```python
from build123d import *

# Parameters (mm, degrees)
F1_R   = 13.7541
F1_R_2 = 10.6807


with BuildPart() as f3:
    # F3: sweep along a path in F2
    with BuildLine(Plane.XY) as f3_path:
        Line((45.4025, 13.7541), (25.0317, 13.7541))
        ThreePointArc((25.0317, 13.7541), (7.3316151854, 6.4224848146), (0, -11.2776))
        Line((0, -11.2776), (0, -31.6484))
    # F1 (on offset) → F3 (sweep)
    with BuildSketch(Plane.XZ.offset(31.6484)):
        Circle(F1_R)
        Circle(F1_R_2, mode=Mode.SUBTRACT)
    sweep(path=f3_path.line)


solid = f3.part
```
Check sheet for the modelled part. Datum: model origin and axes. Units: mm. A direction names the side the tool comes from. Coordinates: 2 decimals unless noted, no trailing zeros. Write each loop counter-clockwise with the first axis right and the second up, starting at its lowest first coordinate (ties: lowest second). Pieces come first, ordered by that corner, then holes. Notation, with made-up numbers: M 15,3 L 31,3 A32 cw 31,29 Z; hole C 29.25,77.25 d8. An arc over 180 degrees is marked long. Write item = value, one per line. Start each with the question number.
1. Sectioned sample at C-C (y = -22). Record the cut outline in (x, z), then the cut area to 3 significant figures.
2. Sectioned sample at A-A (z = 0). Record the cut outline in (x, y), then the cut area to 3 significant figures.
3. Tool access check on faces 4 (the cylindrical face through (9.866, -21.606, -4.091)), 5 (the flat face through (-7.1, -31.648, 8.2)), 6 (the cylindrical face through (35.075, 0.635, 4.131)). Record the directions out of +Z, -Z, +X, -X, +Y, -Y that give a thin tool (end or side, any length) a straight path to the whole face; none if there is none.
4. Sectioned sample at D-D (z = -3.5). Record the cut outline in (x, y).
5. Thickness scan on probe 1 along Z at (x, y) = (0, -26.5); probe 2 along Z at (x, y) = (12.5, 11); probe 3 along Y at (x, z) = (29.5, -5.75). Record the ranges inside material, lowest first.
6. Go/stop test with flat-tipped pins: pin 1 (1 mm diameter, centred on y = 11, z = -1.5, fed in from +X); pin 2 (1 mm diameter, centred on x = 37.5, z = 6, fed in from -Y); pin 3 (2 mm diameter, centred on x = 37, z = 7.5, fed in from +Y). Record where each tip stops, or that it passes through.
7. Sectioned sample at B-B (x = 40). Record the cut outline in (y, z), then the cut area to 3 significant figures.
8. Mould release check, pull along Z, two halves, no side actions. Record for faces 1 (the flat face through (45.402, 20.82, 8.21)), 2 (the cylindrical face through (-13.74, -21.61, 0.6)), 3 (the cylindrical face through (35.07, 22.23, -6.5)): pulls with the +Z half, pulls with the -Z half, needs draft (parallel to the pull), parting line crosses it, or undercut.
The answers:
q1.outline = C 0,0 d27.51; hole C 0,0 d21.36
q1.area = 236 mm²
q2.outline = M -13.75,-31.65 L -10.68,-31.65 L -10.68,-11.28 A35.71 cw 25.03,24.43 L 45.4,24.43 L 45.4,27.51 L 25.03,27.51 A38.79 ccw -13.75,-11.28 Z; M 10.68,-31.65 L 13.75,-31.65 L 13.75,-11.28 A11.28 cw 25.03,0 L 45.4,0 L 45.4,3.07 L 25.03,3.07 A14.35 ccw 10.68,-11.28 Z
q2.area = 492 mm²
q3.face_4 = -Y
q3.face_5 = +Z, -Z, +X, -X, -Y
q3.face_6 = +X
q4.outline = M -13.3,-31.65 L -10.09,-31.65 L -10.09,-11.28 A35.12 cw 25.03,23.85 L 45.4,23.85 L 45.4,27.06 L 25.03,27.06 A38.33 ccw -13.3,-11.28 Z; M 10.09,-31.65 L 13.3,-31.65 L 13.3,-11.28 A11.73 cw 25.03,0.45 L 45.4,0.45 L 45.4,3.66 L 25.03,3.66 A14.94 ccw 10.09,-11.28 Z
q5.probe_1 = -13.75 to -10.68, 10.68 to 13.75
q5.probe_2 = -13.74 to -10.67, 10.67 to 13.74
q5.probe_3 = 1.26 to 4.75, 22.75 to 26.25
q6.pin_1 = -2.33
q6.pin_2 = 1.15
q6.pin_3 = 25.88
q7.outline = C 13.75,0 d27.51; hole C 13.75,0 d21.36
q7.area = 236 mm²
q8.face_1 = needs draft
q8.face_2 = parting line crosses it
q8.face_3 = undercut
